Build history of the part. All positions in model axes, mm. A direction names the side the tool comes from. Give positions to 0.01 mm unless a question says otherwise; leave off trailing zeros. Loops run counter-clockwise (first coordinate to the right, second up) from the corner with the lowest first, then second, coordinate; pieces in that order, holes last.
1) Band-saw the part on B-B on x = 75. List the corners of the cut face in (y, z).
2) Two-plate mould, pull along X, no slides. Class faces 3 (the cylindrical face through (1, 21, -2)), 4 (the cylindrical face through (102.86, 22.52, -69.9)), 5 (the flat face through (115, 20, -44)), 6 (the flat face through (3, 23, -45)): +X half, -X half, draft (parallel to the pull), parting line (faces both ways), or undercut.
3) 3-axis set-ups, long thin cutter, end or side, ignore diameter. For faces 1 (the flat face through (57, 20, -90)), 2 (the flat face through (8, 22, -69)): which of +Z, -Z, +X, -X, +Y, -Y reach the whole face in a straight line?
4) Band-saw the part on C-C on z = -52. List the corners of the cut face in (x, y).
5) Flat gauge pin, fed straight in: P1, Ø6, axis at x = 46, z = -21, coming from the +Y side. Where does the tip first touch, or does it go through?
6) Wall check: line 1 (X direction, y = 27.5, z = -33); line 2 (Z direction, x = 93.5, y = 22.5); line 3 (X direction, y = 13, z = -10). Give the ranges that are in metal, low to high.
```python
from build123d import *

# Parameters (mm, degrees)
SKETCH1_W           = 115
SKETCH1_H           = 90
BOSS_EXTRUDE1_DEPTH = 41.5
SKETCH3_W           = 109
SKETCH3_H           = 84
CUT_EXTRUDE1_DEPTH  = 38.5
SKETCH4_W           = 10
SKETCH4_H           = 18
BOSS_EXTRUDE2_DEPTH = 38.5
FILLET1_R           = 3
FILLET2_R           = 5


with BuildPart() as part:
    # Sketch1 → Boss-Extrude1 (new body)
    with BuildSketch(Plane(origin=(0, 0, 0), x_dir=(1, 0, 0), z_dir=(0, 1, 0))):
        with Locations((57.5, 45)):
            Rectangle(SKETCH1_W, SKETCH1_H)
    extrude(amount=BOSS_EXTRUDE1_DEPTH)

    # Sketch3 → Cut-Extrude1 (cut)
    with BuildSketch(Plane(origin=(0, 41.5, 0), x_dir=(1, 0, 0), z_dir=(0, 1, 0))):
        with Locations((57.5, 45)):
            Rectangle(SKETCH3_W, SKETCH3_H)
    extrude(amount=-CUT_EXTRUDE1_DEPTH, mode=Mode.SUBTRACT)

    # Sketch4 → Boss-Extrude2 (add)
    with BuildSketch(Plane(origin=(0, 3, 0), x_dir=(1, 0, 0), z_dir=(0, 1, 0))):
        with Locations((8, 78)):
            Rectangle(SKETCH4_W, SKETCH4_H)
        with Locations((107, 78)):
            Rectangle(SKETCH4_W, SKETCH4_H)
        with Locations((107, 12)):
            Rectangle(SKETCH4_W, SKETCH4_H)
        with Locations((8, 12)):
            Rectangle(SKETCH4_W, SKETCH4_H)
    extrude(amount=BOSS_EXTRUDE2_DEPTH)

    # Fillet1
    fillet1_edges = [part.edges().sort_by_distance(p)[0] for p in [
        (13, 22.25, -87),
        (13, 22.25, -69),
        (3, 22.25, -69),
        (102, 22.25, -69),
        (102, 22.25, -87),
        (112, 22.25, -69),
        (102, 22.25, -21),
        (112, 22.25, -21),
        (102, 22.25, -3),
        (13, 22.25, -21),
        (13, 22.25, -3),
        (3, 22.25, -21),
    ]]
    fillet(fillet1_edges, radius=FILLET1_R)

    # Fillet2
    fillet2_edges = [part.edges().sort_by_distance(p)[0] for p in [
        (0, 20.75, -90),
        (115, 20.75, -90),
        (115, 20.75, 0),
        (0, 20.75, 0),
    ]]
    fillet(fillet2_edges, radius=FILLET2_R)


solid = part.part
```
Findings below:
1. outline: (0, -90) - (41.5, -90) - (41.5, -87) - (3, -87) - (3, -3) - (41.5, -3) - (41.5, 0) - (0, 0) - close
2. face 3: -X half
2. face 4: undercut
2. face 5: +X half
2. face 6: undercut
3. face 1: -Z, +X, -X, +Y, -Y
3. face 2: +Y
4. outline: (0, 0) - (115, 0) - (115, 41.5) - (112, 41.5) - (112, 3) - (3, 3) - (3, 41.5) - (0, 41.5) - close
5. P1: stops at y = 3
6. line 1: x = 0 to 3, 112 to 115
6. line 2: z = -90 to -87, -3 to 0
6. line 3: x = 0 to 13, 102 to 115
